Build history of the part. All positions in model axes, mm. A direction names the side the tool comes from. Give positions to 0.01 mm unless a question says otherwise; leave off trailing zeros. Order: outer loops, then holes, each group sorted by start corner. A loop starts at its lowest first (then second) coordinate and runs counter-clockwise, first axis right, second up. Notation, with made-up numbers: (36, -40) -> (92, -40) arc R11 ccw to (92, -21) -> close; hole circle Ø2 at (87, 60.5). An arc over 180 degrees is marked (long way). One line per question, with ' | ' between items. Start each with the question number.
(1) Cut at D-D (z = 13.5). Give the cut face in (x, y) (3 decimals).
(2) Cut at C-C (x = -10.5). Give the cut face in (y, z) (3 decimals).
(3) Cut at B-B (y = -9). Give the cut face in (x, z).
(4) Which spindle directions (+Z, -Z, +X, -X, +Y, -Y) get a long thin tool onto all of the face, cutting with end or side? Do faces 5 (the face through (-21.5, -1, 7)), 6 (the face through (0, -15.625, 5)), 7 (the face through (-20.1, -3, 12)). Say none if no direction does.
(5) Pull direction X, two halves, no side cores. Call faces 1 (the face through (0, -1, 0)), 2 (the face through (18.93, 11.774, 4.958)), 3 (the face through (20.93, 14.524, 7.605)), 4 (the face through (-20.899, -16.305, 7.605)): +X half, -X half, draft (parallel to the pull), parting line (faces both ways), or undercut.
(6) Drill centre lines: L1, parallel to X at y = -3, z = 6.5; L2, parallel to X at y = -2.5, z = 9.75; L3, parallel to Y at x = -10, z = 3 (3 decimals). Where is each one in solid material? Low to high. Write a range as from..to.
(7) Pin check, flat tips, straight feed: pin 1 Ø9 at (x, y) = (-5.5, -4.5) entering from +Z; pin 2 Ø1.5 at (x, z) = (9.5, 10) entering from -Y (3 decimals). Stop position of each tip, or through.
(8) Cut at A-A (z = 5.25). Give the cut face in (x, y) (3 decimals), then the cut area to 3 significant figures.
from build123d import *

# Parameters (mm, degrees)
SKETCH1_W           = 43
SKETCH1_H           = 32
BOSS_EXTRUDE1_DEPTH = 15
SKETCH2_W           = 40.2
SKETCH2_H           = 30
CUT_EXTRUDE1_DEPTH  = 7
SKETCH3_W           = 39
SKETCH3_H           = 28
CUT_EXTRUDE2_DEPTH  = 6
FILLET2_R           = 2
FILLET4_R           = 2


with BuildPart() as part:
    # Sketch1 → Boss-Extrude1 (new body)
    with BuildSketch(Plane.XY):
        with Locations((0, -0.875)):
            Rectangle(SKETCH1_W, SKETCH1_H)
    extrude(amount=BOSS_EXTRUDE1_DEPTH)

    # Sketch2 → Cut-Extrude1 (cut)
    with BuildSketch(Plane.XY.offset(15)):
        with Locations((0, -1.875)):
            Rectangle(SKETCH2_W, SKETCH2_H)
    extrude(amount=-CUT_EXTRUDE1_DEPTH, mode=Mode.SUBTRACT)

    # Sketch3 → Cut-Extrude2 (cut)
    with BuildSketch(Plane.XY.offset(8)):
        with Locations((0, -1.625)):
            Rectangle(SKETCH3_W, SKETCH3_H)
    extrude(amount=-CUT_EXTRUDE2_DEPTH, mode=Mode.SUBTRACT)

    # Fillet2
    fillet2_edges = [part.edges().sort_by_distance(p)[0] for p in [
        (20.1, 13.125, 11.5),
        (-20.1, 13.125, 11.5),
        (19.5, 12.375, 5),
        (19.5, -15.625, 5),
        (-19.5, -15.625, 5),
        (-19.5, 12.375, 5),
    ]]
    fillet(fillet2_edges, radius=FILLET2_R)

    # Fillet4
    fillet4_edges = [part.edges().sort_by_distance(p)[0] for p in [
        (-21.5, -16.875, 7.5),
        (21.5, -16.875, 7.5),
        (21.5, 15.125, 7.5),
        (-21.5, 15.125, 7.5),
    ]]
    fillet(fillet4_edges, radius=FILLET4_R)


solid = part.part
Result set:
1) outline: (-21.5, -14.875) arc R2 ccw to (-20.1, -16.783) -> (-20.1, 11.125) arc R2 cw to (-18.1, 13.125) -> (18.1, 13.125) arc R2 cw to (20.1, 11.125) -> (20.1, -16.783) arc R2 ccw to (21.5, -14.875) -> (21.5, 13.125) arc R2 ccw to (19.5, 15.125) -> (-19.5, 15.125) arc R2 ccw to (-21.5, 13.125) -> close
2) outline: (-16.875, 0) -> (15.125, 0) -> (15.125, 15) -> (13.125, 15) -> (13.125, 8) -> (12.375, 8) -> (12.375, 2) -> (-15.625, 2) -> (-15.625, 8) -> (-16.875, 8) -> close
3) outline: (-21.5, 0) -> (21.5, 0) -> (21.5, 15) -> (20.1, 15) -> (20.1, 8) -> (19.5, 8) -> (19.5, 2) -> (-19.5, 2) -> (-19.5, 8) -> (-20.1, 8) -> (-20.1, 15) -> (-21.5, 15) -> close
4) face 5: +Z, -Z, -X, +Y, -Y | face 6: +Z | face 7: +Z, -Y
5) face 1: draft | face 2: undercut | face 3: +X half | face 4: -X half
6) L1: x = -21.5..-19.5, 19.5..21.5 | L2: x = -21.5..-20.1, 20.1..21.5 | L3: y = -16.875..-15.625, 12.375..15.125
7) pin 1: stops at z = 2 | pin 2: stops at y = 13.125
8) outline: (-21.5, -14.875) arc R2 ccw to (-19.5, -16.875) -> (19.5, -16.875) arc R2 ccw to (21.5, -14.875) -> (21.5, 13.125) arc R2 ccw to (19.5, 15.125) -> (-19.5, 15.125) arc R2 ccw to (-21.5, 13.125) -> close; hole (-19.5, -13.625) arc R2 ccw to (-17.5, -15.625) -> (17.5, -15.625) arc R2 ccw to (19.5, -13.625) -> (19.5, 10.375) arc R2 ccw to (17.5, 12.375) -> (-17.5, 12.375) arc R2 ccw to (-19.5, 10.375) -> close | area: 284 mm2
